Input: part model. Units: mm. Frame: model coordinates. A direction names the side the tool comes from. Give positions to 0.01 mm unless a question says otherwise; leave off trailing zeros. Loops run counter-clockwise (first coordinate to the right, second up) from the corner with the lowest first, then second, coordinate; pieces in that order, holes last.
from build123d import *

# Parameters (mm, degrees)
SKETCH1_R                = 15
SKETCH1_R_2              = 13.5
BOSS_EXTRUDE1_DEPTH      = 250
SKETCH2_R                = 15
BOSS_EXTRUDE2_DEPTH      = 5
SKETCH3_R                = 15
SKETCH3_R_2              = 7
BOSS_EXTRUDE3_DEPTH      = 5
SKETCH4_W                = 20
SKETCH4_H                = 15
SKETCH4_R                = 2.5
BOSS_EXTRUDE4_DEPTH      = 10
BOSS_EXTRUDE4_DEPTH_BACK = 10
SKETCH5_W                = 14
SKETCH5_H                = 15
CUT_EXTRUDE1_DEPTH       = 20


with BuildPart() as part:
    # Sketch1 → Boss-Extrude1 (new body)
    with BuildSketch(Plane.XY):
        Circle(SKETCH1_R)
        Circle(SKETCH1_R_2, mode=Mode.SUBTRACT)
    extrude(amount=BOSS_EXTRUDE1_DEPTH)

    # Sketch2 → Boss-Extrude2 (add)
    with BuildSketch(Plane(origin=(0, 0, 0), x_dir=(-1, 0, 0), z_dir=(0, 0, -1))):
        Circle(SKETCH2_R)
    extrude(amount=BOSS_EXTRUDE2_DEPTH)

    # Sketch3 → Boss-Extrude3 (add)
    with BuildSketch(Plane.XY.offset(250)):
        Circle(SKETCH3_R)
        Circle(SKETCH3_R_2, mode=Mode.SUBTRACT)
    extrude(amount=BOSS_EXTRUDE3_DEPTH)

    # Sketch4 → Boss-Extrude4 (add, two sides)
    with BuildSketch(Plane(origin=(0, 0, 0), x_dir=(0, 0, -1), z_dir=(1, 0, 0))) as boss_extrude4_sk:
        with Locations((15, 0)):
            Rectangle(SKETCH4_W, SKETCH4_H)
        with Locations((20, 0)):
            Circle(SKETCH4_R, mode=Mode.SUBTRACT)
    extrude(amount=BOSS_EXTRUDE4_DEPTH)
    extrude(boss_extrude4_sk.sketch, amount=-BOSS_EXTRUDE4_DEPTH_BACK)

    # Sketch5 → Cut-Extrude1 (cut)
    with BuildSketch(Plane(origin=(0, 0, -25), x_dir=(-1, 0, 0), z_dir=(0, 0, -1))):
        Rectangle(SKETCH5_W, SKETCH5_H)
    extrude(amount=-CUT_EXTRUDE1_DEPTH, mode=Mode.SUBTRACT)


solid = part.part
(1) Cut plane D-D (z = 19). Return the cut outline in (x, y), and give its area (3 significant figures).
Values follow:
outline: circle Ø30 at (0, 0); hole circle Ø27 at (0, 0)
area: 134 mm2
(2) Pin query (flat end, axial travel): pin 1 Ø8 at (y, z) = (7, 214.5) entering from -X; pin 2 Ø4.5 at (y, z) = (2, -15.5) entering from -X; pin 3 Ø2.5 at (x, z) = (-9, -19) entering from +Y. Return the tip coordinate at first contact, or that it passes through.
Values follow:
pin 1: stops at x = -14.7
pin 2: stops at x = -10
pin 3: stops at y = 7.5
(3) Mould query, pull axis Y, two halves, no side actions, for faces 1 (the cylindrical face through (-8.5, 0.1, -17.5)), 2 (the cylindrical face through (-2.93, -13.18, 123.25)), 3 (the flat face through (10, 0, -15)). Classes: +Y half, -Y half, draft (parallel to the pull), parting line (faces both ways), or undercut.
Values follow:
face 1: undercut
face 2: undercut
face 3: draft
(4) Reachability of faces 4 (the flat face through (-10, 0, -15)), 5 (the flat face through (6, -6, 250)), 6 (the cylindrical face through (6.466, -2.681, 252.465)), 7 (the cylindrical face through (8.5, 0.1, -17.5)), 8 (the flat face through (7, 0, -15)) from +Z, -Z, +X, -X, +Y, -Y: full face, straight path, thin tool, end or side. Return the list, or none.
Values follow:
face 4: -Z, -X, +Y, -Y
face 5: none
face 6: +Z
face 7: +X, -X
face 8: -Z, +Y, -Y
(5) Cut plane A-A (z = -20). Return the cut outline in (x, y).
Values follow:
outline: (-10, -7.5) - (-7, -7.5) - (-7, -2.5) - (-10, -2.5) - close; (-10, 2.5) - (-7, 2.5) - (-7, 7.5) - (-10, 7.5) - close; (7, -7.5) - (10, -7.5) - (10, -2.5) - (7, -2.5) - close; (7, 2.5) - (10, 2.5) - (10, 7.5) - (7, 7.5) - close
(6) Cut plane C-C (x = 0). Return the cut outline in (y, z).
Values follow:
outline: (-15, -5) - (15, -5) - (15, 255) - (7, 255) - (7, 250) - (13.5, 250) - (13.5, 0) - (-13.5, 0) - (-13.5, 250) - (-7, 250) - (-7, 255) - (-15, 255) - close
(7) Cut plane B-B (y = 0). Return the cut outline in (x, z).
Values follow:
outline: (-15, -5) - (-10, -5) - (-10, -17.5) - (-7, -17.5) - (-7, -5) - (7, -5) - (7, -17.5) - (10, -17.5) - (10, -5) - (15, -5) - (15, 255) - (7, 255) - (7, 250) - (13.5, 250) - (13.5, 0) - (-13.5, 0) - (-13.5, 250) - (-7, 250) - (-7, 255) - (-15, 255) - close; (-10, -25) - (-7, -25) - (-7, -22.5) - (-10, -22.5) - close; (7, -25) - (10, -25) - (10, -22.5) - (7, -22.5) - close
(8) Ray query, probe 1 along Y at (x, z) = (9.2, -20); probe 2 along Z at (x, y) = (8, 0); probe 3 along Z at (x, y) = (-5, -5.5). Return the intervals inside material, ascending.
Values follow:
probe 1: y = -7.5 to -2.5, 2.5 to 7.5
probe 2: z = -25 to -22.5, -17.5 to 0, 250 to 255
probe 3: z = -5 to 0, 250 to 255
